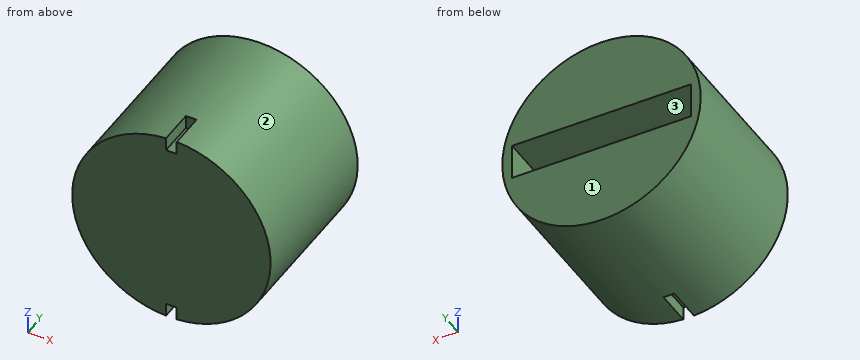
```python
from build123d import *

# Parameters (mm, degrees)
SKETCH1_R           = 13.875
BOSS_EXTRUDE1_DEPTH = 22
SKETCH2_W           = 1.5
SKETCH2_H           = 2.924695476
SKETCH2_H_2         = 4.466803309
CUT_EXTRUDE1_DEPTH  = 5
SKETCH3_W           = 25
SKETCH3_H           = 5
CUT_EXTRUDE2_DEPTH  = 20


with BuildPart() as part:
    # Sketch1 → Boss-Extrude1 (new body)
    with BuildSketch(Plane(origin=(0, 0, 0), x_dir=(1, 0, 0), z_dir=(0, 1, 0))):
        with Locations(Location((0, 0, 0), (0, 0, 270))):
            Circle(SKETCH1_R)
    extrude(amount=BOSS_EXTRUDE1_DEPTH)

    # Sketch2 → Cut-Extrude1 (cut)
    with BuildSketch(Plane.XZ):
        with Locations((0, 13.462347738)):
            Rectangle(SKETCH2_W, SKETCH2_H)
        with Locations((0, -14.233401654)):
            Rectangle(SKETCH2_W, SKETCH2_H_2)
    extrude(amount=-CUT_EXTRUDE1_DEPTH, mode=Mode.SUBTRACT)

    # Sketch3 → Cut-Extrude2 (cut)
    with BuildSketch(Plane(origin=(0, 22, 0), x_dir=(1, 0, 0), z_dir=(0, 1, 0))):
        Rectangle(SKETCH3_W, SKETCH3_H)
    extrude(amount=-CUT_EXTRUDE2_DEPTH, mode=Mode.SUBTRACT)


solid = part.part
```
Check sheet for the modelled part. Datum: model origin and axes. Units: mm. Face numbers are marked on the shaded views. Give positions to 0.01 mm unless a question says otherwise; leave off trailing zeros. Write each loop counter-clockwise with the first axis right and the second up, starting at its lowest first coordinate (ties: lowest second). Pieces come first, ordered by that corner, then holes. Notation, with made-up numbers: (83, 20) - (129, 20) arc R4 cw to (129, 26) - close; hole circle Ø8 at (36.5, 41). An arc over 180 degrees is marked (long way). Answer as a JSON object with one key per item and string values. Group by question number.
1) Sectioned sample at A-A (x = 0). Record the cut outline in (y, z) (3 decimals).
2) Release check for a two-part mould opening along X. For the marked faces 1, 2 and 3 record: pulls with the +X half, pulls with the -X half, needs draft (parallel to the pull), parting line crosses it, or undercut.
3) Thickness scan on probe 1 along X at (y, z) = (4.5, -0.5); probe 2 along Z at (x, y) = (9.25, 15.25); probe 3 along Y at (x, z) = (10.25, -2). Record the ranges inside material, lowest first. Write a range as from..to.
4) Sectioned sample at C-C (z = 0). Record the cut outline in (x, y) (3 decimals), then the cut area to 4 significant figures.
5) Depth check by flat-ended pin: P1, Ø1.6, axis at x = 0, y = 2.5, coming from the +Z side; P2, Ø6, axis at x = -10, y = 5.5, coming from the -Z side; P3, Ø5, axis at y = 5, z = -4.5, coming from the +X side; P4, Ø10, axis at y = 14, z = 1, coming from the -X side (3 decimals). Enter the tip coordinate at first touch or a pass-through.
6) Sectioned sample at B-B (y = 15.75). Record the cut outline in (x, z) (3 decimals), then the cut area to 3 significant figures.
7) Sectioned sample at D-D (x = -8). Record the cut outline in (y, z), then the cut area to 3 significant figures.
Geometry results:
{
 "1": {"outline": "(0, -12) - (5, -12) - (5, -13.875) - (22, -13.875) - (22, -2.5) - (2, -2.5) - (2, 2.5) - (22, 2.5) - (22, 13.875) - (5, 13.875) - (5, 12) - (0, 12) - close"},
 "2": {"face 1": "needs draft", "face 2": "parting line crosses it", "face 3": "undercut"},
 "3": {"probe 1": "x = -13.87..-12.5, 12.5..13.87", "probe 2": "z = -10.34..-2.5, 2.5..10.34", "probe 3": "y = 0..2"},
 "4": {"outline": "(-13.875, 0) - (13.875, 0) - (13.875, 22) - (12.5, 22) - (12.5, 2) - (-12.5, 2) - (-12.5, 22) - (-13.875, 22) - close", "area": "110.5 mm^2"},
 "5": {"P1": "stops at z = 13.85", "P2": "stops at z = -11.98", "P3": "stops at x = 13.73", "P4": "stops at x = -13.875"},
 "6": {"outline": "circle Ø27.75 at (0, 0); hole (-12.5, -2.5) - (12.5, -2.5) - (12.5, 2.5) - (-12.5, 2.5) - close", "area": "480 mm^2"},
 "7": {"outline": "(0, -11.34) - (22, -11.34) - (22, -2.5) - (2, -2.5) - (2, 2.5) - (22, 2.5) - (22, 11.34) - (0, 11.34) - close", "area": "399 mm^2"}
}
